Read the model definition and answer for the solid it produces. Units are mm, in the model's axes. A direction names the side the tool comes from. Coordinates: 2 decimals unless noted, no trailing zeros. Write each loop counter-clockwise with the first axis right and the second up, starting at its lowest first coordinate (ties: lowest second). Pieces come first, ordered by that corner, then holes. Notation, with made-up numbers: (47.5, 14) -> (103.5, 14) arc R21 cw to (103.5, 21) -> close; hole circle Ø9 at (-5.5, 51.25). An arc over 180 degrees is marked (long way). Return JSON: item names as keys, results as strings.
from build123d import *

# Parameters (mm, degrees)
BOSS_EXTRUDE1_DEPTH     = 50
SKETCH2_R               = 9
CUT_EXTRUDE1_DEPTH      = 26
CUT_EXTRUDE1_DEPTH_BACK = 181
SKETCH3_W               = 60
SKETCH3_H               = 42
CUT_EXTRUDE2_DEPTH      = 15
SKETCH4_R               = 3
SKETCH4_R_2             = 4
CUT_EXTRUDE3_DEPTH      = 21
SKETCH4_3_R             = 7.5
CUT_EXTRUDE4_DEPTH      = 5


with BuildPart() as part:
    # Sketch1 → Boss-Extrude1 (new body, symmetric)
    with BuildSketch(Plane.XY):
        Polygon((0, 0), (0, 15), (-25, 15), (-25, 85), (-45, 85), (-45, 35), (-105, 35), (-105, 20), (-205, 20), (-205, 0), align=None)
    extrude(amount=BOSS_EXTRUDE1_DEPTH, both=True)

    # Sketch2 → Cut-Extrude1 (cut, two sides)
    with BuildSketch(Plane(origin=(-25, 0, 0), x_dir=(0, 0, -1), z_dir=(1, 0, 0))) as cut_extrude1_sk:
        with Locations((0, 45)):
            Circle(SKETCH2_R)
    extrude(amount=CUT_EXTRUDE1_DEPTH, mode=Mode.SUBTRACT)
    extrude(cut_extrude1_sk.sketch, amount=-CUT_EXTRUDE1_DEPTH_BACK, mode=Mode.SUBTRACT)

    # Sketch3 → Cut-Extrude2 (cut)
    with BuildSketch(Plane(origin=(0, 35, 0), x_dir=(1, 0, 0), z_dir=(0, 1, 0))):
        with Locations((-75, 0)):
            Rectangle(SKETCH3_W, SKETCH3_H)
    extrude(amount=-CUT_EXTRUDE2_DEPTH, mode=Mode.SUBTRACT)

    # Sketch4 → Cut-Extrude3 (cut, through all)
    with BuildSketch(Plane(origin=(0, 20, 0), x_dir=(1, 0, 0), z_dir=(0, 1, 0))):
        with Locations((-182.5, 17)):
            Circle(SKETCH4_R)
        with Locations((-123, 35)):
            Circle(SKETCH4_R_2)
        with Locations((-12.5, 35)):
            Circle(SKETCH4_R_2)
        with Locations((-12.5, -35)):
            Circle(SKETCH4_R_2)
        with Locations((-123, -35)):
            Circle(SKETCH4_R_2)
        with Locations((-182.5, -17)):
            Circle(SKETCH4_R)
    extrude(amount=-CUT_EXTRUDE3_DEPTH, mode=Mode.SUBTRACT)

    # Sketch4_3 → Cut-Extrude4 (cut)
    with BuildSketch(Plane(origin=(0, 20, 0), x_dir=(1, 0, 0), z_dir=(0, 1, 0))):
        with Locations((-123, 35)):
            Circle(SKETCH4_3_R)
        with Locations((-12.5, 35)):
            Circle(SKETCH4_3_R)
        with Locations((-12.5, -35)):
            Circle(SKETCH4_3_R)
        with Locations((-123, -35)):
            Circle(SKETCH4_3_R)
    extrude(amount=-CUT_EXTRUDE4_DEPTH, mode=Mode.SUBTRACT)


solid = part.part
1. The part is cut by section C-C (y = 45). Determine the outline of the cut face in (x, z).
Taken from the geometry:
{"outline": "(-45, -50) -> (-25, -50) -> (-25, -9) -> (-45, -9) -> close; (-45, 9) -> (-25, 9) -> (-25, 50) -> (-45, 50) -> close"}
2. Consider L1, parallel to Z at x = -12.5, y = 11; L2, parallel to X at y = 11, z = -35; L3, parallel to Z at x = -123, y = 18.6. Determine where each line is inside the solid, lowest interval first.
Taken from the geometry:
{"L1": "z = -50 to -39, -31 to 31, 39 to 50", "L2": "x = -205 to -127, -119 to -16.5, -8.5 to 0", "L3": "z = -50 to -42.5, -27.5 to 27.5, 42.5 to 50"}
3. For a pull along Z with two mould halves and no side action, classify faces 1 (the face through (-12, 15, 1)), 2 (the face through (-13.021, 7.605, 31.034)), 3 (the face through (-81, 24, 50)) as +Z half, -Z half, draft (parallel to the pull), parting line (faces both ways), or undercut.
Taken from the geometry:
{"face 1": "draft", "face 2": "undercut", "face 3": "+Z half"}
4. A tool of negligible diameter and unlimited length cuts with its end or side. For faces 4 (the face through (-75, 28, 21)), 5 (the face through (-75, 35, 36)), 6 (the face through (-120, 15, -32)), from which of +Z, -Z, +X, -X, +Y, -Y can it reach the whole face along a straight path? Write none if from no direction.
Taken from the geometry:
{"face 4": "-X, +Y", "face 5": "+Z, -Z, -X, +Y", "face 6": "+Y"}
5. The part is cut by section D-D (z = 0). Determine the outline of the cut face in (x, y).
Taken from the geometry:
{"outline": "(-205, 0) -> (0, 0) -> (0, 15) -> (-25, 15) -> (-25, 36) -> (-45, 36) -> (-45, 20) -> (-205, 20) -> close; (-45, 54) -> (-25, 54) -> (-25, 85) -> (-45, 85) -> close"}
6. The part is cut by section A-A (x = -182.5). Determine the outline of the cut face in (y, z), then the cut area to 3 significant figures.
Taken from the geometry:
{"outline": "(0, -50) -> (20, -50) -> (20, -20) -> (0, -20) -> close; (0, -14) -> (20, -14) -> (20, 14) -> (0, 14) -> close; (0, 20) -> (20, 20) -> (20, 50) -> (0, 50) -> close", "area": "1,760 mm2"}
7. Flat-ended cylindrical pins translate along their axes: pin 1 Ø4.5 at (x, z) = (-122, 33) entering from +Y; pin 2 Ø4 at (y, z) = (28, 10) entering from +X; pin 3 Ø23 at (x, z) = (-64.5, 37.5) entering from +Y; pin 4 Ø6.5 at (x, z) = (-123, 35) entering from +Y. Find the tip coordinate at first contact, or state that the pin passes through.
Taken from the geometry:
{"pin 1": "stops at y = 15", "pin 2": "stops at x = -25", "pin 3": "stops at y = 35", "pin 4": "passes through"}
8. The part is cut by section B-B (z = 35). Determine the outline of the cut face in (x, y), then the cut area to 3 significant figures.
Taken from the geometry:
{"outline": "(-205, 0) -> (-127, 0) -> (-127, 15) -> (-130.5, 15) -> (-130.5, 20) -> (-205, 20) -> close; (-119, 0) -> (-16.5, 0) -> (-16.5, 15) -> (-25, 15) -> (-25, 85) -> (-45, 85) -> (-45, 35) -> (-105, 35) -> (-105, 20) -> (-115.5, 20) -> (-115.5, 15) -> (-119, 15) -> close; (-8.5, 0) -> (0, 0) -> (0, 15) -> (-8.5, 15) -> close", "area": "5,860 mm2"}
